Build history of the part. All positions in model axes, mm. Face numbers are marked on the shaded views. A direction names the side the tool comes from. Round coordinates to 2 decimals unless told otherwise and drop trailing zeros. Write each loop counter-clockwise with the first axis right and the second up, starting at its lowest first coordinate (ties: lowest second). Pieces come first, ordered by that corner, then holes. Notation, with made-up numbers: M 26,47 L 53,47 A18 cw 53,79 Z; hole C -22.75,73 d2. An arc over 180 degrees is marked long. Use a Markdown table: item, result.
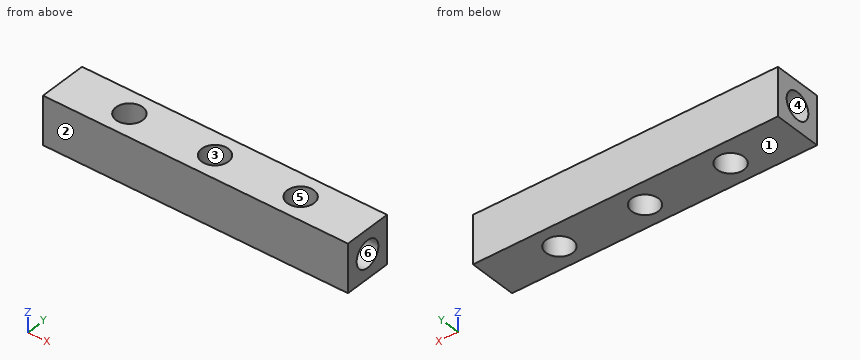
from build123d import *

# Parameters (mm, degrees)
SKETCH1_W                      = 28.5
SKETCH1_H                      = 4.5
BOSS_EXTRUDE1_DEPTH            = 4.5
SIDE_SHAFT_HOLES_M3_AT_2_COUNT = 2
SIDE_SHAFT_HOLES_M3_AT_2_PITCH = 47.562875198
M3X0_5_TAPPED_HOLE3_D          = 2.5


with BuildPart() as part:
    # Sketch1 → Boss-Extrude1 (new body)
    with BuildSketch(Plane.XY):
        with Locations((-14.25, 37.5)):
            Rectangle(SKETCH1_W, SKETCH1_H)
    extrude(amount=BOSS_EXTRUDE1_DEPTH)

    # Sketch2 → Side Shaft Holes (M3) (revolve, cut)
    with BuildSketch(Plane(origin=(0, 37.5, 2.25), x_dir=(0, 0, -1), z_dir=(0, 1, 0))):
        Polygon((0, 0), (0, 4), (1.25, 3.248924226), (1.25, 0), align=None)
    side_shaft_holes_m3 = revolve(axis=Axis((6.35, 37.5, 2.25), (-1, 0, 0)), mode=Mode.SUBTRACT)

    # Side Shaft Holes (M3) at 2: Side Shaft Holes (M3) ×2
    with Locations(*[(0, 0, -i * SIDE_SHAFT_HOLES_M3_AT_2_PITCH) for i in range(1, SIDE_SHAFT_HOLES_M3_AT_2_COUNT)]):
        add(side_shaft_holes_m3, mode=Mode.SUBTRACT)

    # Shaft Hole Mirror: Side Shaft Holes (M3) across plane
    add(side_shaft_holes_m3.mirror(Plane.ZY.offset(14.25)), mode=Mode.SUBTRACT)

    # Shaft Hole Mirror copy 1 sketch → Shaft Hole Mirror copy 1 (revolve, cut)
    with BuildSketch(Plane(origin=(-28.5, 37.5, -45.312875198), x_dir=(0, 0, -1), z_dir=(0, 1, 0))):
        Polygon((0, 0), (0, -4), (1.25, -3.248924226), (1.25, 0), align=None)
    revolve(axis=Axis((-34.85, 37.5, -45.312875198), (-1, 0, 0)), mode=Mode.SUBTRACT)

    # M3x0.5 Tapped Hole3 (through all)
    with Locations(Plane.XY.offset(4.5)):
        with Locations((-6.25, 37.5), (-14.25, 37.5), (-22.25, 37.5)):
            Hole(M3X0_5_TAPPED_HOLE3_D / 2)


solid = part.part
Q1. Drill centre lines: L1, parallel to Y at x = -6.25, z = 2.4; L2, parallel to Z at x = -27.35, y = 37.5; L3, parallel to X at y = 38.3, z = 0.85. Where is each one in solid material? Low to high.
Response values:
| item | result |
|---|---|
| L1 | y = 35.25 to 36.25, 38.75 to 39.75 |
| L2 | z = 0 to 1, 3.5 to 4.5 |
| L3 | x = -28.5 to -23.21, -21.29 to -15.21, -13.29 to -7.21, -5.29 to 0 |
Q2. Which spindle directions (+Z, -Z, +X, -X, +Y, -Y) get a long thin tool onto all of the face, cutting with end or side? Do the marked faces 4, 5 and 6. Say none if no direction does.
Response values:
| item | result |
|---|---|
| face 4 | -X |
| face 5 | +Z, -Z |
| face 6 | +X |
Q3. Drop a flat-ended pin along its axis: P1, Ø2, axis at y = 37.5, z = 2.25, coming from the -X side. Give the stop position or say it passes through.
Response values:
| item | result |
|---|---|
| P1 | stops at x = -25.1 |
Q4. Cut at A-A on x = -6.25. Give the cut face in (y, z), and give its area (3 significant figures).
Response values:
| item | result |
|---|---|
| outline | M 35.25,0 L 36.25,0 L 36.25,4.5 L 35.25,4.5 Z; M 38.75,0 L 39.75,0 L 39.75,4.5 L 38.75,4.5 Z |
| area | 9.00 mm2 |
Q5. Cut at B-B on y = 37.05. Count the separate pieces of the cut face and the enclosed holes in it, and give its area (3 significant figures).
Response values:
| item | result |
|---|---|
| separate pieces | 4 |
| enclosed holes | 0 |
| area | 80.3 mm2 |
Q6. Cut at C-C on x = -22. Give the cut face in (y, z).
Response values:
| item | result |
|---|---|
| outline | M 35.25,0 L 36.28,0 L 36.28,4.5 L 35.25,4.5 Z; M 38.72,0 L 39.75,0 L 39.75,4.5 L 38.72,4.5 Z |
Q7. Two-plate mould, pull along Y, no slides. Class the marked faces 1, 2 and 3: +Y half, -Y half, draft (parallel to the pull), parting line (faces both ways), or undercut.
Response values:
| item | result |
|---|---|
| face 1 | draft |
| face 2 | -Y half |
| face 3 | undercut |
